The listing builds one solid part. Answer for the finished solid, in the listing's coordinates (mm). A direction names the side the tool comes from. Give positions to 0.01 mm unless a question says otherwise; leave off trailing zeros. Loops run counter-clockwise (first coordinate to the right, second up) from the corner with the lowest first, then second, coordinate; pieces in that order, holes last. Notation, with made-up numbers: M 24.25,79 L 46.25,79 A22 cw 46.25,95 Z; hole C 4,77 d1. An arc over 180 degrees is marked long. Use one line per item in the form item = value. Start each with the question number.
1. Each of these flat-tipped pins is pushed along its axis until it touches: pin 1 Ø4 at (x, y) = (0.5, 6) entering from +Z; pin 2 Ø10 at (x, y) = (0, -11.13) entering from +Z; pin 3 Ø1.6 at (x, z) = (0, 22.5) entering from +Y; pin 4 Ø2 at (y, z) = (-16, 9.5) entering from +X. Where does it stop, or does it pass through?
2. The part is cut by section C-C (y = -0.25). Write down the section's boundary in (x, z), and give its area (3 significant figures).
3. The part is cut by section D-D (x = 0). Write down the section's boundary in (y, z), and give its area (3 significant figures).
4. The mould has two halves that part along Y. Classify faces 6 (the face through (4, -5, 0)), 7 (the face through (8.496, -18.156, 15.21)), 8 (the face through (-6.2, -1, 15)), 9 (the face through (0, 1.353, 15)): released by +Y, released by -Y, zero draft, split by the parting line, or undercut.
5. For faces 1 (the face through (5.214, 5.984, 16.818)), 2 (the face through (-0.6, -18.5, 8.3)), 3 (the face through (4, -5, 30)), 4 (the face through (0, -3.606, 15)), 5 (the face through (-10, -3, 15)), determine the directions among +Z, -Z, +X, -X, +Y, -Y from which every point of the face is accessible in a straight line to the end or side of a thin tool.
6. The part is cut by section B-B (x = 3.5). Write down the section's boundary in (y, z).
7. Straight lines are drawn through the part: line 1 (Z direction, x = 0, y = -18.8); line 2 (Y direction, x = 0, z = 10); line 3 (X direction, y = -0.5, z = 23.5). For each, find the intervals that lie inside material, in ascending order. Write a range as from..to.
8. The part is cut by section A-A (z = 7.5). Write down the section's boundary in (x, y), and give its area (3 significant figures).
from build123d import *

# Parameters (mm, degrees)
ESBO_O1_W                = 4.958931368
ESBO_O1_H                = 12.4
RESSALTO_EXTRUS_O1_DEPTH = 30
RESSALTO_EXTRUS_O2_DEPTH = 4
FILETE1_R                = 5
ESBO_O3_R                = 1
CORTE_EXTRUS_O1_DEPTH    = 4


with BuildPart() as part:
    # Esboço1 → Ressalto-extrusão1 (new body)
    with BuildSketch(Plane(origin=(0, 0, 0), x_dir=(0, 1, 0), z_dir=(0, 0, 1))):
        Polygon((3.617797035, 6.2), (3.617797035, -6.2), (8.417797035, -4.2), (8.417797035, -10), (-11.126254615, -10), (-19.582202965, -10), (-19.582202965, 10), (-11.126254615, 10), (8.417797035, 10), (8.417797035, 4.2), align=None)
        with Locations((-1.126254615, 0)):
            Rectangle(ESBO_O1_W, ESBO_O1_H, mode=Mode.SUBTRACT)
        with BuildLine():
            ThreePointArc((-11.126254615, -6.35), (-4.776254615, 0), (-11.126254615, 6.35))
            ThreePointArc((-11.126254615, 6.35), (-17.476254615, 0), (-11.126254615, -6.35))
        make_face(mode=Mode.SUBTRACT)
    extrude(amount=RESSALTO_EXTRUS_O1_DEPTH)

    # Esboço2 → Ressalto-extrusão2 (add)
    with BuildSketch(Plane(origin=(0, 0, 0), x_dir=(0, 1, 0), z_dir=(0, 0, 1))):
        Polygon((8.417797035, -4.2), (3.617797035, -6.2), (3.617797035, 6.2), (8.417797035, 4.2), align=None)
    extrude(amount=RESSALTO_EXTRUS_O2_DEPTH)

    # Filete1
    filete1_edges = [part.edges().sort_by_distance(p)[0] for p in [
        (10, -19.582202965, 15),
        (-10, -19.582202965, 15),
    ]]
    fillet(filete1_edges, radius=FILETE1_R)

    # Esboço3 → Corte-extrusão1 (cut)
    with BuildSketch(Plane.XZ.offset(19.582202965)):
        with Locations(Location((0, 22.5, 0), (0, 0, 270))):
            Circle(ESBO_O3_R)
        with Locations(Location((0, 7.5, 0), (0, 0, 270))):
            Circle(ESBO_O3_R)
    extrude(amount=-CORTE_EXTRUS_O1_DEPTH, mode=Mode.SUBTRACT)


solid = part.part
Derived:
q1.pin_1 = 4
q1.pin_2 = through
q1.pin_3 = 3.62
q1.pin_4 = 9.98
q2.outline = M -10,0 L -6.2,0 L -6.2,30 L -10,30 Z; M 6.2,0 L 10,0 L 10,30 L 6.2,30 Z
q2.area = 228 mm2
q3.outline = M -19.58,0 L -17.48,0 L -17.48,6.5 L -19.58,6.5 Z; M -19.58,8.5 L -17.48,8.5 L -17.48,21.5 L -19.58,21.5 Z; M -19.58,23.5 L -17.48,23.5 L -17.48,30 L -19.58,30 Z; M -4.78,0 L -3.61,0 L -3.61,30 L -4.78,30 Z; M 1.35,0 L 8.42,0 L 8.42,4 L 3.62,4 L 3.62,30 L 1.35,30 Z
q3.area = 177 mm2
q4.face_6 = zero draft
q4.face_7 = released by -Y
q4.face_8 = undercut
q4.face_9 = undercut
q5.face_1 = +Z
q5.face_2 = -Y
q5.face_3 = +Z, +X, -X, +Y, -Y
q5.face_4 = +Z, -Z
q5.face_5 = +Z, -Z, -X, +Y, -Y
q6.outline = M -19.58,0 L -16.42,0 L -16.42,30 L -19.58,30 Z; M -5.83,0 L -3.61,0 L -3.61,30 L -5.83,30 Z; M 1.35,0 L 8.42,0 L 8.42,4 L 3.62,4 L 3.62,30 L 1.35,30 Z
q7.line_1 = 0..6.5, 8.5..21.5, 23.5..30
q7.line_2 = -19.58..-17.48, -4.78..-3.61, 1.35..3.62
q7.line_3 = -10..-6.2, 6.2..10
q8.outline = M -10,-14.58 A5 ccw -5,-19.58 L -1,-19.58 L -1,-17.4 A6.35 cw long 1,-17.4 L 1,-19.58 L 5,-19.58 A5 ccw 10,-14.58 L 10,8.42 L 4.2,8.42 L 6.2,3.62 L -6.2,3.62 L -4.2,8.42 L -10,8.42 Z; hole M -6.2,-3.61 L 6.2,-3.61 L 6.2,1.35 L -6.2,1.35 Z
q8.area = 307 mm2
